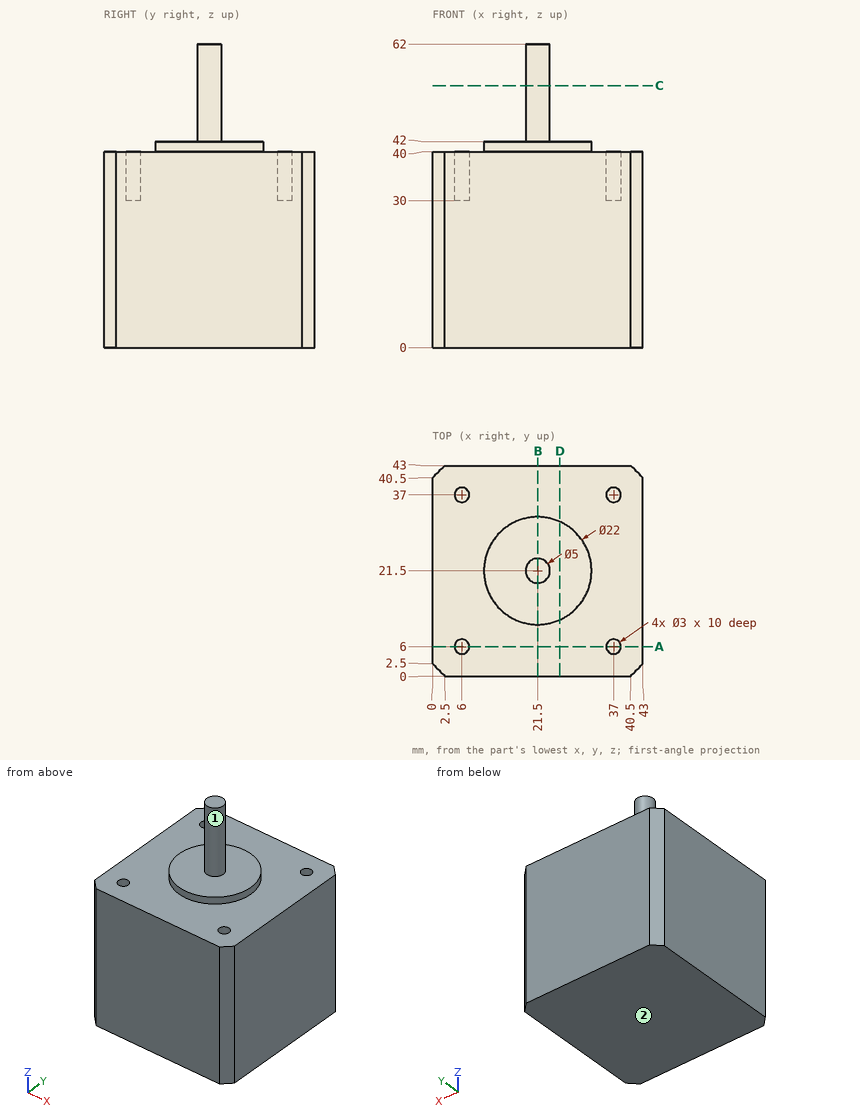
Design review of the part shown in the three views and the two pictorial views. Dimensions are in mm from the part's minimum x, y and z. A direction names the side the tool comes from. Round coordinates to 2 decimals unless told otherwise and drop trailing zeros. Loops run counter-clockwise (first coordinate to the right, second up) from the corner with the lowest first, then second, coordinate; pieces in that order, holes last.
1) Consider section A-A on y = 6. State the section outline as (x, z) points, then the cut area to 3 significant figures.
Values follow:
outline: (0, 0) - (43, 0) - (43, 40) - (38.5, 40) - (38.5, 30) - (35.5, 30) - (35.5, 40) - (7.5, 40) - (7.5, 30) - (4.5, 30) - (4.5, 40) - (0, 40) - close
area: 1,660 mm2
2) Tool access review of the marked faces 1 and 2: name each direction out of +Z, -Z, +X, -X, +Y, -Y from which nothing blocks a thin tool from reaching the whole face with its end or side.
Values follow:
face 1: +Z
face 2: -Z, +X, -X, +Y, -Y
3) Consider section B-B on x = 21.5. State the section outline as (y, z) points.
Values follow:
outline: (0, 0) - (43, 0) - (43, 40) - (32.5, 40) - (32.5, 42) - (24, 42) - (24, 62) - (19, 62) - (19, 42) - (10.5, 42) - (10.5, 40) - (0, 40) - close
4) Consider section C-C on z = 53.5. State the section outline as (x, y) points, then the cut area to 3 significant figures.
Values follow:
outline: circle Ø5 at (21.5, 21.5)
area: 19.6 mm2
5) Clearance check with flat-ended pins moving along their axes: P1, Ø3.5, axis at x = 5.5, y = 6.5, coming from the +Z side; P2, Ø17.5, axis at x = 17, y = 22.5, coming from the +Z side; P3, Ø1.5, axis at x = 6, y = 37.5, coming from the +Z side; P4, Ø5, axis at x = 26.5, y = 16, coming from the +Z side. State where each tip first meets the part, or that it passes through.
Values follow:
P1: stops at z = 40
P2: stops at z = 62
P3: stops at z = 30
P4: stops at z = 42
6) Wall thickness on line 1 along Y through (x, z) = (37, 36); line 2 along Z through (x, y) = (38, 9.5); line 3 along Z through (x, y) = (37, 37): over which ranges is each line inside the solid? List them lowest first.
Values follow:
line 1: y = 0 to 4.5, 7.5 to 35.5, 38.5 to 43
line 2: z = 0 to 40
line 3: z = 0 to 30
7) Consider section D-D on x = 26. State the section outline as (y, z) points, then the cut area to 3 significant figures.
Values follow:
outline: (0, 0) - (43, 0) - (43, 40) - (31.54, 40) - (31.54, 42) - (11.46, 42) - (11.46, 40) - (0, 40) - close
area: 1,760 mm2
